The model under review builds one solid part; all positions refer to its coordinate system, in mm. Give positions to 0.01 mm unless a question says otherwise; leave off trailing zeros. Loops run counter-clockwise (first coordinate to the right, second up) from the corner with the lowest first, then second, coordinate; pieces in that order, holes last. Notation, with made-up numbers: (15, 46.5) - (51, 46.5) arc R22 ccw to (51, 81.5) - close; hole circle Ø7 at (23.25, 72.5). An arc over 180 degrees is marked (long way). Return JSON: item names as keys, results as strings. Group by question number.
```python
from build123d import *

# Parameters (mm, degrees)
SKETCH2_R                 = 11.5
BOSS_EXTRUDE1_DEPTH       = 80
CHAMFER1_SIZE             = 1
M6X1_0_TAPPED_HOLE1_D     = 5
M6X1_0_TAPPED_HOLE1_DEPTH = 11.5
M6X1_0_TAPPED_HOLE1_TIP   = 1.502151548


with BuildPart() as part:
    # Sketch2 → Boss-Extrude1 (new body)
    with BuildSketch(Plane.XY):
        Circle(SKETCH2_R)
    extrude(amount=BOSS_EXTRUDE1_DEPTH)

    # Chamfer1
    chamfer1_edges = [part.edges().sort_by_distance(p)[0] for p in [
        (-11.5, 0, 0),
        (-11.5, 0, 80),
    ]]
    chamfer(chamfer1_edges, length=CHAMFER1_SIZE)

    # M6x1.0 Tapped Hole1
    with Locations(Plane.XZ.offset(11.5)):
        with Locations((0, 15)):
            Hole(M6X1_0_TAPPED_HOLE1_D / 2, depth=M6X1_0_TAPPED_HOLE1_DEPTH)
            with Locations((0, 0, -(M6X1_0_TAPPED_HOLE1_DEPTH + M6X1_0_TAPPED_HOLE1_TIP / 2))):  # 118° drill point
                Cone(0, M6X1_0_TAPPED_HOLE1_D / 2, M6X1_0_TAPPED_HOLE1_TIP, mode=Mode.SUBTRACT)


solid = part.part
```
1) For pin 1 Ø4 at (y, z) = (5.5, 26.5) entering from +X; pin 2 Ø1.5 at (x, z) = (-5.5, 35.5) entering from -Y; pin 3 Ø1.5 at (x, z) = (-7.5, 24.5) entering from +Y, all flat-tipped, find the tip position at first contact; note any pin that passes through.
2) Draft analysis for pull direction X (two halves, no side actions). For faces 1 (the face through (-1.5, 11.4, 39.5)), 2 (the face through (0, 0, 80)), 3 (the face through (0.54, -5.67, 12.56)), state which applies: +X half, -X half, draft (parallel to the pull), parting line (faces both ways), or undercut.
3) We need section A-A, the plane z = 31. Write out the cut boundary in (x, y).
4) To check wall thickness, follow line 1 (Z direction, x = 0, y = -6.75); line 2 (Y direction, x = 0, z = 62.5); line 3 (X direction, y = -7.25, z = 15). State the ranges of each line that lie inside material, in increasing order.
Findings:
{
 "1": {"pin 1": "stops at x = 10.95", "pin 2": "stops at y = -10.47", "pin 3": "stops at y = 9.31"},
 "2": {"face 1": "parting line", "face 2": "draft", "face 3": "undercut"},
 "3": {"outline": "circle Ø23 at (0, 0)"},
 "4": {"line 1": "z = 0 to 12.5, 17.5 to 80", "line 2": "y = -11.5 to 11.5", "line 3": "x = -8.93 to -2.5, 2.5 to 8.93"}
}
